from build123d import *

# Parameters (mm, degrees)
SKETCH1_W           = 48
SKETCH1_H           = 25
BOSS_EXTRUDE1_DEPTH = 4
SKETCH2_W           = 30
SKETCH2_H           = 25
BOSS_EXTRUDE2_DEPTH = 15
SKETCH3_R           = 1.5
CUT_EXTRUDE1_DEPTH  = 20
SKETCH4_R           = 1.6
CUT_EXTRUDE2_DEPTH  = 20


with BuildPart() as part:
    # Sketch1 → Boss-Extrude1 (new body)
    with BuildSketch(Plane(origin=(0, 0, 0), x_dir=(1, 0, 0), z_dir=(0, 1, 0))):
        Rectangle(SKETCH1_W, SKETCH1_H)
    extrude(amount=BOSS_EXTRUDE1_DEPTH)

    # Sketch2 → Boss-Extrude2 (add)
    with BuildSketch(Plane(origin=(0, 4, 0), x_dir=(1, 0, 0), z_dir=(0, 1, 0))):
        Rectangle(SKETCH2_W, SKETCH2_H)
    extrude(amount=BOSS_EXTRUDE2_DEPTH)

    # Sketch3 → Cut-Extrude1 (cut, through all)
    with BuildSketch(Plane(origin=(0, 19, 0), x_dir=(1, 0, 0), z_dir=(0, 1, 0))):
        with Locations(Location((0, 7.975, 0), (0, 0, 270))):  # turned: the seam where the file's is
            Circle(SKETCH3_R)
        with Locations(Location((0, -7.975, 0), (0, 0, 270))):  # turned: the seam where the file's is
            Circle(SKETCH3_R)
        with Locations(Location((-11, 7.5, 0), (0, 0, 270))):  # turned: the seam where the file's is
            Circle(SKETCH3_R)
        with Locations(Location((-11, -7.5, 0), (0, 0, 270))):  # turned: the seam where the file's is
            Circle(SKETCH3_R)
    extrude(amount=-CUT_EXTRUDE1_DEPTH, mode=Mode.SUBTRACT)

    # Sketch4 → Cut-Extrude2 (cut, through all)
    with BuildSketch(Plane.XZ):
        with Locations(Location((-20, 9, 0), (0, 0, 270))):  # turned: the seam where the file's is
            Circle(SKETCH4_R)
        with Locations(Location((20, 9, 0), (0, 0, 270))):  # turned: the seam where the file's is
            Circle(SKETCH4_R)
        with Locations(Location((20, -9, 0), (0, 0, 270))):  # turned: the seam where the file's is
            Circle(SKETCH4_R)
        with Locations(Location((-20, -9, 0), (0, 0, 270))):  # turned: the seam where the file's is
            Circle(SKETCH4_R)
    extrude(amount=-CUT_EXTRUDE2_DEPTH, mode=Mode.SUBTRACT)


solid = part.part
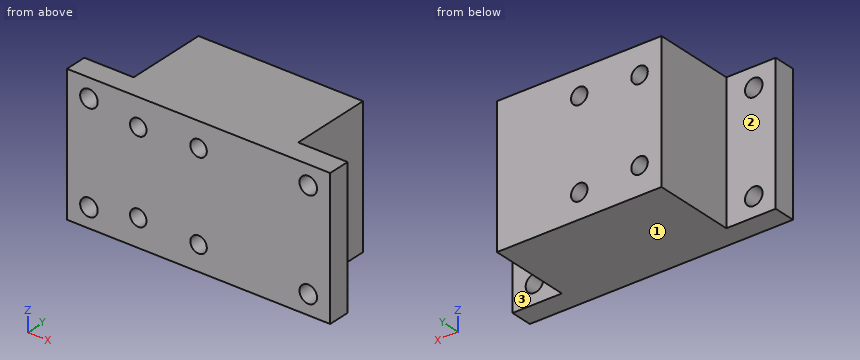
Model file for the job. Use its own axes, mm. Face numbers are marked on the shaded views. A direction names the side the tool comes from. Give positions to 0.01 mm unless a question says otherwise; leave off trailing zeros. Order: outer loops, then holes, each group sorted by start corner. A loop starts at its lowest first (then second) coordinate and runs counter-clockwise, first axis right, second up. Notation, with made-up numbers: (46.25, -32.5) - (95.25, -32.5) arc R15 cw to (95.25, -21.5) - close; hole circle Ø2 at (-10, 3). An arc over 180 degrees is marked (long way). Write item = value, one per line. Start each with the question number.
1. Probe line 1 along X through (y, z) = (10, -7.5); line 2 along X through (y, z) = (7.5, -8.75); line 3 along X through (y, z) = (16.75, 3). List the from-to ranges inside material, lowest first.
2. Cut at C-C, the plane z = -3. List the corners of the cut face in (x, y).
3. Which spindle directions (+Z, -Z, +X, -X, +Y, -Y) get a long thin tool onto all of the face, cutting with end or side? Do the marked faces 1, 2 and 3. Say none if no direction does.
4. Drop flat-ended pins along their axis: P1, Ø7, axis at x = -19.5, z = 0, coming from the +Y side; P2, Ø4, axis at y = 8, z = -5.5, coming from the +X side; P3, Ø1.8, axis at x = 0, z = 7.975, coming from the -Y side. Give the stop position or say it passes through.
5. Cut at D-D, the plane y = 3. State how many separate pieces and enclosed holes the cut face has, and give its area (3 significant figures).
6. Cut at B-B, the plane y = 12.5. List the corners of the cut face in (x, z) (3 decimals).
7. Cut at A-A, the plane x = -20. List the corners of the cut face in (y, z), and give its area (3 significant figures).
Taken from the geometry:
q1.line_1 = -15 to -12.5, -9.5 to -1.42, 1.42 to 15
q1.line_2 = -15 to -11.83, -10.17 to -1.28, 1.28 to 15
q1.line_3 = -15 to 15
q2.outline = (-24, 0) - (24, 0) - (24, 4) - (15, 4) - (15, 19) - (-15, 19) - (-15, 4) - (-24, 4) - close
q3.face_1 = -Z, +X, -X, +Y, -Y
q3.face_2 = +Z, -Z, -X, +Y
q3.face_3 = +Z, -Z, +X, +Y
q4.P1 = 4
q4.P2 = 15
q4.P3 = through
q5.separate_pieces = 1
q5.enclosed_holes = 8
q5.area = 1,140 mm²
q6.outline = (-15, -12.5) - (15, -12.5) - (15, 12.5) - (-15, 12.5) - close; hole circle Ø3 at (-11, -7.5); hole circle Ø3 at (-11, 7.5); hole circle Ø3 at (0, -7.975); hole circle Ø3 at (0, 7.975)
q7.outline = (0, -12.5) - (4, -12.5) - (4, -10.6) - (0, -10.6) - close; (0, -7.4) - (4, -7.4) - (4, 7.4) - (0, 7.4) - close; (0, 10.6) - (4, 10.6) - (4, 12.5) - (0, 12.5) - close
q7.area = 74.4 mm²
